Read the model definition and answer for the solid it produces. Units are mm, in the model's axes. A direction names the side the tool comes from. Coordinates: 2 decimals unless noted, no trailing zeros. Write each loop counter-clockwise with the first axis right and the second up, starting at its lowest first coordinate (ties: lowest second). Pieces come first, ordered by that corner, then holes. Notation, with made-up numbers: (63, 30) -> (100, 30) arc R12 ccw to (100, 47) -> close; hole circle Ø11 at (52, 39). An arc over 180 degrees is marked (long way). Answer in a Markdown table with one row per item. Add a question column.
Item 1: For a pull along Y with two mould halves and no side action, classify faces 1 (the face through (22, -46.8, -3)), 2 (the face through (29.178, -43, -3)), 3 (the face through (22, -47.308, -3)), 4 (the face through (21.7, -46.5, 0)) as +Y half, -Y half, draft (parallel to the pull), parting line (faces both ways), or undercut.
Item 2: Section D-D on x = 15.5 is taken. Write down the section's boundary in (y, z).
Item 3: Which of the six approach directions +Z, -Z, +X, -X, +Y, -Y give full straight-line access (tool end or side, diameter ignored) to faces 5 (the face through (22, -47, -4.762)), 6 (the face through (22.3, -46.6, -0.762))?
Item 4: Straight lines are drawn through the part: line 1 (X direction, y = -41.75, z = -0.4); line 2 (Y direction, x = 28.75, z = -3.6); line 3 (X direction, y = -44.5, z = -3.3). For each, find the intervals that lie inside material, in ascending order. Write a range as from..to.
Item 5: Section B-B on z = -0.6 is taken. Write down the section's boundary in (x, y).
Item 6: Section A-A on y = -45.5 is taken. Write down the section's boundary in (x, z), then the cut area to 3 significant figures.
Item 7: Section C-C on x = 23 is taken. Write down the section's boundary in (y, z).
```python
from build123d import *

# Parameters (mm, degrees)
SKETCH1_W           = 14.9225
SKETCH1_H           = 8.255
SKETCH1_W_2         = 12.8905
SKETCH1_H_2         = 6.223
BOSS_EXTRUDE1_DEPTH = 4.7625
SKETCH2_W           = 13.9065
SKETCH2_H           = 7.239
CUT_EXTRUDE1_DEPTH  = 4.0005
FILLET1_R           = 0.381


with BuildPart() as part:
    # Sketch1 → Boss-Extrude1 (new body)
    with BuildSketch(Plane.XY):
        with Locations((22.225, -43.18)):
            Rectangle(SKETCH1_W, SKETCH1_H)
        with Locations((22.225, -43.18)):
            Rectangle(SKETCH1_W_2, SKETCH1_H_2, mode=Mode.SUBTRACT)
    extrude(amount=-BOSS_EXTRUDE1_DEPTH)

    # Sketch2 → Cut-Extrude1 (cut)
    with BuildSketch(Plane(origin=(0, 0, -4.7625), x_dir=(-1, 0, 0), z_dir=(0, 0, -1))):
        with Locations((-22.225, -43.18)):
            Rectangle(SKETCH2_W, SKETCH2_H)
    extrude(amount=-CUT_EXTRUDE1_DEPTH, mode=Mode.SUBTRACT)

    # Fillet1
    fillet1_edges = [part.edges().sort_by_distance(p)[0] for p in [
        (22.225, -47.3075, 0),
        (14.76375, -43.18, 0),
        (22.225, -39.0525, 0),
        (29.68625, -43.18, 0),
        (29.68625, -47.3075, -2.38125),
        (14.76375, -47.3075, -2.38125),
        (14.76375, -39.0525, -2.38125),
        (29.68625, -39.0525, -2.38125),
    ]]
    fillet(fillet1_edges, radius=FILLET1_R)


solid = part.part
```
Results below:
| question | item | result |
|---|---|---|
| 1 | face 1 | undercut |
| 1 | face 2 | undercut |
| 1 | face 3 | -Y half |
| 1 | face 4 | draft |
| 2 | outline | (-47.31, -4.76) -> (-46.8, -4.76) -> (-46.8, -0.76) -> (-39.56, -0.76) -> (-39.56, -4.76) -> (-39.05, -4.76) -> (-39.05, -0.38) arc R0.38 ccw to (-39.43, 0) -> (-46.93, 0) arc R0.38 ccw to (-47.31, -0.38) -> close |
| 3 | face 5 | -Z, +X, -X, +Y, -Y |
| 3 | face 6 | -Z |
| 4 | line 1 | x = 14.76..15.78, 28.67..29.69 |
| 4 | line 2 | y = -47.31..-46.8, -39.56..-39.05 |
| 4 | line 3 | x = 14.76..15.27, 29.18..29.69 |
| 5 | outline | (14.76, -46.93) arc R0.38 ccw to (15.14, -47.31) -> (29.31, -47.31) arc R0.38 ccw to (29.69, -46.93) -> (29.69, -39.43) arc R0.38 ccw to (29.31, -39.05) -> (15.14, -39.05) arc R0.38 ccw to (14.76, -39.43) -> close; hole (15.78, -46.29) -> (28.67, -46.29) -> (28.67, -40.07) -> (15.78, -40.07) -> close |
| 6 | outline | (14.76, -4.76) -> (15.27, -4.76) -> (15.27, -0.76) -> (15.78, -0.76) -> (15.78, 0) -> (15.14, 0) arc R0.38 ccw to (14.76, -0.38) -> close; (28.67, -0.76) -> (29.18, -0.76) -> (29.18, -4.76) -> (29.69, -4.76) -> (29.69, -0.38) arc R0.38 ccw to (29.31, 0) -> (28.67, 0) -> close |
| 6 | area | 5.55 mm2 |
| 7 | outline | (-47.31, -4.76) -> (-46.8, -4.76) -> (-46.8, -0.76) -> (-46.29, -0.76) -> (-46.29, 0) -> (-46.93, 0) arc R0.38 ccw to (-47.31, -0.38) -> close; (-40.07, -0.76) -> (-39.56, -0.76) -> (-39.56, -4.76) -> (-39.05, -4.76) -> (-39.05, -0.38) arc R0.38 ccw to (-39.43, 0) -> (-40.07, 0) -> close |
